The model under review builds one solid part; all positions refer to its coordinate system, in mm. A direction names the side the tool comes from. Round coordinates to 2 decimals unless told otherwise and drop trailing zeros. Loops run counter-clockwise (first coordinate to the right, second up) from the corner with the lowest first, then second, coordinate; pieces in that order, holes last. Notation, with made-up numbers: M 13.25,2.25 L 54.25,2.25 A17 ccw 54.25,21.25 Z; hole C 22,48 d11. An arc over 180 degrees is marked long. Use a Markdown table: item, result. Add a question column.
```python
from build123d import *

# Parameters (mm, degrees)
SKETCH1_W           = 23.75
SKETCH1_H           = 24
BOSS_EXTRUDE1_DEPTH = 10
SKETCH2_W           = 3.3
SKETCH2_H           = 9.8
BOSS_EXTRUDE2_DEPTH = 23.75
SKETCH3_W           = 3.3
SKETCH3_H           = 17.3
SKETCH3_H_2         = 3.35
SKETCH3_H_3         = 13.15
BOSS_EXTRUDE3_DEPTH = 4.9
CUT_EXTRUDE1_REACH  = 36.413
SKETCH4_R           = 1.9
SKETCH5_W           = 3.5
SKETCH5_H           = 17.5
SKETCH5_H_2         = 3.25
SKETCH5_H_3         = 13.05
CUT_EXTRUDE2_DEPTH  = 5


with BuildPart() as part:
    # Sketch1 → Boss-Extrude1 (new body)
    with BuildSketch(Plane.YZ):
        with Locations((11.875, 12)):
            Rectangle(SKETCH1_W, SKETCH1_H)
    extrude(amount=-BOSS_EXTRUDE1_DEPTH)

    # Sketch2 → Boss-Extrude2 (add, through all)
    with BuildSketch(Plane.XZ):
        with Locations((-5, -4.9)):
            Rectangle(SKETCH2_W, SKETCH2_H)
    extrude(amount=-BOSS_EXTRUDE2_DEPTH)

    # Sketch3 → Boss-Extrude3 (add)
    with BuildSketch(Plane.XZ):
        with Locations((-5, 12)):
            Rectangle(SKETCH3_W, SKETCH3_H)
        with Locations((-5, 22.325)):
            Rectangle(SKETCH3_W, SKETCH3_H_2)
        with Locations((-5, -3.225)):
            Rectangle(SKETCH3_W, SKETCH3_H_3)
    extrude(amount=BOSS_EXTRUDE3_DEPTH)

    # Sketch4 → Cut-Extrude1 (cut, up to next)
    with BuildSketch(Plane(origin=(-6.65, 0, 0), x_dir=(0, -1, 0), z_dir=(-1, 0, 0)), mode=Mode.PRIVATE) as cut_extrude1_sk1:
        with Locations(Location((-11.875, -5, 0), (0, 0, 90))):
            Circle(SKETCH4_R)
    cut_extrude1_tool1 = extrude(cut_extrude1_sk1.sketch, amount=-CUT_EXTRUDE1_REACH, mode=Mode.PRIVATE) & part.part
    add(cut_extrude1_tool1.solids().sort_by_distance((-6.65, 11.875, -5))[0], mode=Mode.SUBTRACT)

    # Sketch5 → Cut-Extrude2 (cut)
    with BuildSketch(Plane(origin=(0, 23.75, 0), x_dir=(-1, 0, 0), z_dir=(0, 1, 0))):
        with Locations((5, 12)):
            Rectangle(SKETCH5_W, SKETCH5_H)
        with Locations((5, 22.375)):
            Rectangle(SKETCH5_W, SKETCH5_H_2)
        with Locations((5, -3.275)):
            Rectangle(SKETCH5_W, SKETCH5_H_3)
    extrude(amount=-CUT_EXTRUDE2_DEPTH, mode=Mode.SUBTRACT)


solid = part.part
```
(1) Consider section D-D, the plane y = 14.5. Give the boundary of the cut face in (x, z), then the cut area to 3 significant figures.
(2) Insertion check: pin 1 Ø3.5 at (y, z) = (11.875, -5) entering from +X; pin 2 Ø1.5 at (y, z) = (5, -5) entering from -X; pin 3 Ø3.5 at (x, z) = (-8.5, 13) entering from -Y; pin 4 Ø1 at (x, y) = (-2.5, 12.5) entering from -Z. Each pin has a flat end and moves straight along its axis. Give the tip position at first contact, or say it passes through.
(3) To check wall thickness, follow probe 1 along Y at (x, z) = (-4.85, -5) (3 decimals); probe 2 along X at (y, z) = (20.5, 4); probe 3 along Z at (x, y) = (-2.5, 18.5). State the ranges of each line that lie inside material, in increasing order.
(4) For faces 4 (the face through (-8, 12, 0)), 5 (the face through (-2, 12, 0)), 6 (the face through (-8, 0, 12)), 7 (the face through (-6.75, 21, 12)), list the 3-axis set-ups (+Z, -Z, +X, -X, +Y, -Y) from which the entire face can be reached by the end or side of a thin tool; tool diameter is ignored.
(5) Consider section B-B, the plane y = 21.5. Give the boundary of the cut face in (x, z), then the cut area to 3 significant figures.
(6) Consider section C-C, the plane z = 10.5. Give the boundary of the cut face in (x, y), then the cut area to 3 significant figures.
(7) Draft analysis for pull direction Y (two halves, no side actions). For faces 1 (the face through (-2, 0, 12)), 2 (the face through (-5.02, 11.96, -6.9)), 3 (the face through (-10, 12, 12)), state which applies: released by +Y, released by -Y, zero draft, split by the parting line, or undercut.
(8) Consider section A-A, the plane z = -5. Give the boundary of the cut face in (x, y) (3 decimals).
Found:
| question | item | result |
|---|---|---|
| 1 | outline | M -10,0 L -6.65,0 L -6.65,-9.8 L -3.35,-9.8 L -3.35,0 L 0,0 L 0,24 L -10,24 Z |
| 1 | area | 272 mm^2 |
| 2 | pin 1 | passes through |
| 2 | pin 2 | stops at x = -6.65 |
| 2 | pin 3 | stops at y = 0 |
| 2 | pin 4 | stops at z = 0 |
| 3 | probe 1 | y = -4.9 to 9.975, 13.775 to 18.75 |
| 3 | probe 2 | x = -10 to -6.75, -3.25 to 0 |
| 3 | probe 3 | z = 0 to 24 |
| 4 | face 4 | -Z, -X, +Y, -Y |
| 4 | face 5 | -Z, +X, +Y, -Y |
| 4 | face 6 | +Z, -Z, -X, -Y |
| 4 | face 7 | +Z, -Z, +Y |
| 5 | outline | M -10,0 L -6.75,0 L -6.75,24 L -10,24 Z; M -3.25,0 L 0,0 L 0,24 L -3.25,24 Z |
| 5 | area | 156 mm^2 |
| 6 | outline | M -10,0 L -6.65,0 L -6.65,-4.9 L -3.35,-4.9 L -3.35,0 L 0,0 L 0,23.75 L -3.25,23.75 L -3.25,18.75 L -6.75,18.75 L -6.75,23.75 L -10,23.75 Z |
| 6 | area | 236 mm^2 |
| 7 | face 1 | released by -Y |
| 7 | face 2 | undercut |
| 7 | face 3 | zero draft |
| 8 | outline | M -6.65,-4.9 L -3.35,-4.9 L -3.35,9.975 L -6.65,9.975 Z; M -6.65,13.775 L -3.35,13.775 L -3.35,18.75 L -6.65,18.75 Z |
